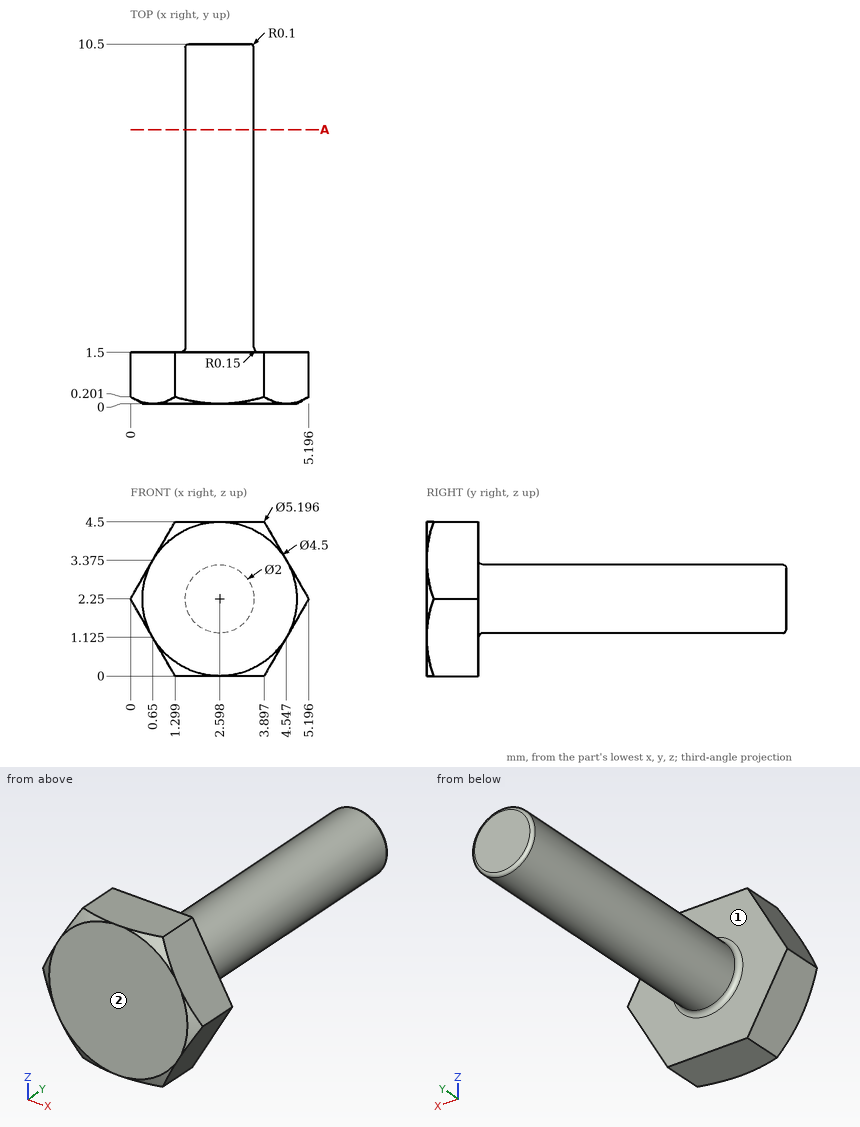
Study the drawing (mm; zero at the part's minimum x, y, z) and answer. A direction names the side the tool comes from. Give positions to 0.01 mm unless a question says otherwise; leave off trailing zeros. Loops run counter-clockwise (first coordinate to the right, second up) from the corner with the lowest first, then second, coordinate; pieces in that order, holes last. Notation, with made-up numbers: M 52,53 L 67,53 A19 ccw 67,88 Z; hole C 79,41 d11. An arc over 180 degrees is marked long. One line per item, written item: value. Start each with the question number.
1. Find the intervals of material crossed by probe 1 along Y at (x, z) = (4.65, 2.35); probe 2 along Z at (x, y) = (2.6, 2.25); probe 3 along X at (y, z) = (5, 2.2), in increasing order.
2. Find section A-A (y = 8). Give the vertices of the cut face in (x, z).
3. Which of the six approach directions +Z, -Z, +X, -X, +Y, -Y give full straight-line access (tool end or side, diameter ignored) to the marked faces 1 and 2?
Reported:
1. probe 1: y = 0 to 1.5
1. probe 2: z = 1.25 to 3.25
1. probe 3: x = 1.6 to 3.6
2. outline: C 2.6,2.25 d2
3. face 1: +Y
3. face 2: +Z, -Z, +X, -X, -Y
